from build123d import *

# Parameters (mm, degrees)
EXTRUDE_1_DEPTH = 3
FILLET_1_R      = 0.381
FILLET_2_R      = 2.032
FILLET_3_R      = 0.508


with BuildPart() as part:
    # 스케치1 → 보스-돌출1 (new body)
    with BuildSketch(Plane.XY):
        with BuildLine():
            ThreePointArc((6.35, 3.529721173), (5.670280833, 0.435941066), (3.756321038, -2.08799463))
            ThreePointArc((3.756321038, -2.08799463), (1.146216202, -5.391882357), (0, -9.443364775))
            ThreePointArc((0, -9.443364775), (-1.146216202, -5.391882357), (-3.756321038, -2.08799463))
            ThreePointArc((-3.756321038, -2.08799463), (-5.670280833, 0.435941066), (-6.35, 3.529721173))
            Line((-6.35, 3.529721173), (-1.4475, 3.529721173))
            Line((-1.4475, 3.529721173), (-1.4475, 0.529721173))
            Line((-1.4475, 0.529721173), (1.4475, 0.529721173))
            Line((1.4475, 0.529721173), (1.4475, 3.529721173))
            Line((1.4475, 3.529721173), (6.35, 3.529721173))
        make_face()
    extrude(amount=EXTRUDE_1_DEPTH)

    # 필렛1
    fillet_1_edges = [part.edges().sort_by_distance(p)[0] for p in [
        (0, -9.443364775, 1.5),
    ]]
    fillet(fillet_1_edges, radius=FILLET_1_R)

    # 필렛2
    fillet_2_edges = [part.edges().sort_by_distance(p)[0] for p in [
        (-6.35, 3.529721173, 1.5),
        (6.35, 3.529721173, 1.5),
    ]]
    fillet(fillet_2_edges, radius=FILLET_2_R)

    # 필렛3
    fillet_3_edges = [part.edges().sort_by_distance(p)[0] for p in [
        (-1.4475, 3.529721173, 1.5),
        (1.4475, 3.529721173, 1.5),
    ]]
    fillet(fillet_3_edges, radius=FILLET_3_R)


solid = part.part
Read the model definition and answer for the solid it produces. Units are mm, in the model's axes. A direction names the side the tool comes from. Coordinates: 2 decimals unless noted, no trailing zeros. Loops run counter-clockwise (first coordinate to the right, second up) from the corner with the lowest first, then second, coordinate; pieces in that order, holes last. Notation, with made-up numbers: (-14, 56) -> (22, 56) arc R11 ccw to (22, 70) -> close; hole circle Ø4 at (-37, 4.5). An arc over 180 degrees is marked (long way). Write item = value, one per line. Start each with the question number.
1) The part is cut by section C-C, the plane x = 3.5. Determine the outline of the cut face in (y, z), plus the area to 3 significant figures.
2) Find the intervals of material crossed by L1, parallel to X at y = 2.75, z = 1.65; L2, parallel to X at y = 2, z = 0.4; L3, parallel to Y at x = -5, z = 0.6, in increasing order. Write a range as from..to.
3) The part is cut by section B-B, the plane y = -5.25. Determine the outline of the cut face in (x, z), plus the area to 3 significant figures.
4) Given P1, Ø1.4, axis at x = 0, z = 2, coming from the +Y side; P2, Ø1.5, axis at x = -2.5, y = -2, coming from the -Z side, each flat-ended and moving along its own axis, determine where each tip first touches the part or whether it passes through.
5) The mould has two halves that part along X. Classify faces 3 (the face through (0, -1, 0)), 4 (the face through (5.62, 2.606, 1.521)), 5 (the face through (0, 0.53, 1)), 6 (the face through (-1.643, -4.522, 1.479)): pulls with the +X half, pulls with the -X half, needs draft (parallel to the pull), parting line crosses it, or undercut.
6) For faces 1 (the face through (-4.93, -0.82, 1.48)), 2 (the face through (1.448, 2, 1)), determine the directions among +Z, -Z, +X, -X, +Y, -Y from which every point of the face is accessible in a straight line to the end or side of a thin tool.
7) The part is cut by section A-A, the plane y = 1.75. Determine the outline of the cut face in (x, z).
Result:
q1.outline = (-2.31, 0) -> (3.53, 0) -> (3.53, 3) -> (-2.31, 3) -> close
q1.area = 17.5 mm²
q2.L1 = -5.52..-1.45, 1.45..5.52
q2.L2 = -5.89..-1.45, 1.45..5.89
q2.L3 = -0.73..3.22
q3.outline = (-1.22, 0) -> (1.22, 0) -> (1.22, 3) -> (-1.22, 3) -> close
q3.area = 7.32 mm²
q4.P1 = 0.53
q4.P2 = 0
q5.face_3 = needs draft
q5.face_4 = pulls with the +X half
q5.face_5 = undercut
q5.face_6 = pulls with the -X half
q6.face_1 = +Z, -Z, -X, -Y
q6.face_2 = +Z, -Z, +Y
q7.outline = (-5.93, 0) -> (-1.45, 0) -> (-1.45, 3) -> (-5.93, 3) -> close; (1.45, 0) -> (5.93, 0) -> (5.93, 3) -> (1.45, 3) -> close
